```python
from build123d import *

# Parameters (mm, degrees)
F0_W     = 145
F0_H     = 70
F1_DEPTH = 2
F2_W     = 5
F2_H     = 2
F3_DEPTH = 3
F4_W     = 5
F4_H     = 2
F5_DEPTH = 3


with BuildPart() as f1:
    # F0 (on Top) → F1 (new body)
    with BuildSketch(Plane.XY):
        with Locations((-24.19392, -13.970558)):
            Rectangle(F0_W, F0_H)
    extrude(amount=F1_DEPTH)

    # F2 (on face) → F3 (join)
    with BuildSketch(Plane(origin=(-96.69392, 0, 0), x_dir=(0, -1, 0), z_dir=(-1, 0, 0))):
        with Locations((-13.529442, 1)):
            Rectangle(F2_W, F2_H)
        with Locations((41.470558, 1)):
            Rectangle(F2_W, F2_H)
    extrude(amount=F3_DEPTH)

    # F4 (on face) → F5 (join)
    with BuildSketch(Plane.YZ.offset(48.30608)):
        with Locations((13.529442, 1)):
            Rectangle(F4_W, F4_H)
        with Locations((-41.470558, 1)):
            Rectangle(F4_W, F4_H)
    extrude(amount=F5_DEPTH)


solid = f1.part
```
Model file for the job. Use its own axes, mm. Give positions to 0.01 mm unless a question says otherwise; leave off trailing zeros. Loops run counter-clockwise (first coordinate to the right, second up) from the corner with the lowest first, then second, coordinate; pieces in that order, holes last. Notation, with made-up numbers: M -33.75,71.25 L 10.25,71.25 A24 cw 10.25,106.25 Z; hole C 57.25,51 d9. An arc over 180 degrees is marked long. Use one line per item in the form item = value.
Item 1: Flat gauge pins, fed straight in: pin 1 Ø0.6 at (x, z) = (-99, 1) entering from +Y; pin 2 Ø1 at (x, z) = (-98, 1) entering from -Y; pin 3 Ø0.6 at (y, z) = (-47.5, 0.5) entering from -X. Where does each tip first touch, or does it go through?
Filled in:
pin_1 = 16.03
pin_2 = -43.97
pin_3 = -96.69
Item 2: Slice it at B-B on y = -2. List the corners of the cut face in (x, z).
Filled in:
outline = M -96.69,0 L 48.31,0 L 48.31,2 L -96.69,2 Z
Item 3: Slice it at A-A on z = 1.15. List the corners of the cut face in (x, y).
Filled in:
outline = M -99.69,-43.97 L -96.69,-43.97 L -96.69,-48.97 L 48.31,-48.97 L 48.31,-43.97 L 51.31,-43.97 L 51.31,-38.97 L 48.31,-38.97 L 48.31,11.03 L 51.31,11.03 L 51.31,16.03 L 48.31,16.03 L 48.31,21.03 L -96.69,21.03 L -96.69,16.03 L -99.69,16.03 L -99.69,11.03 L -96.69,11.03 L -96.69,-38.97 L -99.69,-38.97 Z
Item 4: Drill centre line: L1, parallel to X at y = -16, z = 0.95. Where is it in solid material? Low to high.
Filled in:
L1 = -96.69 to 48.31
